Model file for the job. Use its own axes, mm. Coordinates: 2 decimals unless noted, no trailing zeros. Write each loop counter-clockwise with the first axis right and the second up, starting at its lowest first coordinate (ties: lowest second). Pieces come first, ordered by that corner, then holes.
Q1. Band-saw the part on A-A, the plane x = 50. Write the cut outline in (y, z).
Q2. Band-saw the part on B-B, the plane z = 1.75. State how many separate pieces and enclosed holes the cut face has, plus the area to 3 significant figures.
Q3. Drill centre lines: probe 1 along Y at (x, z) = (-70, 2.25); probe 2 along Z at (x, y) = (-20, 6.75); probe 3 along Y at (x, z) = (-70, 6.25). Where is each one in solid material? Low to high.
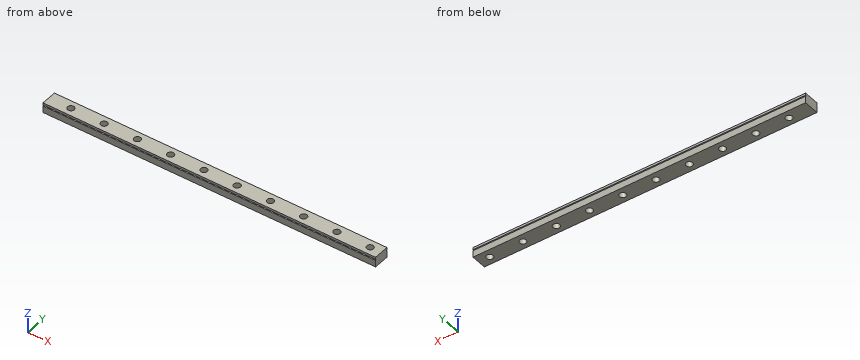
Autodesk Inventor part; units mm, degrees
ref_plane "YZ Plane" through (0, 0, 0) normal (1, 0, 0) x (0, 1, 0)
ref_plane "XZ Plane" through (0, 0, 0) normal (0, 1, 0) x (-1, 0, 0)
ref_plane "XY Plane" through (0, 0, 0) normal (0, 0, 1) x (1, 0, 0)
sketch "Sketch1" plane through (0, 0, 0) normal (0, 0, 1) x (1, 0, 0)
  line L0 (150, -7) -> (-150, -7)
  line L1 (-150, -7) -> (-150, 7)
  line L2 (-150, 7) -> (150, 7)
  line L3 (150, 7) -> (150, -7)
  line L4 (0, 0) -> (0, 3.6651)
  line L5 (0, 0) -> (24.411, 0)
  point P0 (0, 7)
  point P1 (150, 0)
  dimension "d0" = 300
  dimension "d1" = 14
extrude "Extrusion1" add sketch "Sketch1" along normal blind 9
sketch "Sketch2" plane through (-150, -7, 0) normal (-1, 0, 0) x (0, 0, 1)
  line L0 (0, 14) -> (9, 14)
  line L1 (6.5, 13.134) -> (6, 14)
  line L2 (6, 14) -> (7, 14)
  line L3 (7, 14) -> (6.5, 13.134)
  point P0 (0, 7)
  point P1 (6.5, 13.7113)
  dimension "d4" = 1
  dimension "d5" = 2
extrude "Extrusion2" cut sketch "Sketch2" against normal through all
mirror "Mirror1" about plane through (0, 0, 0) normal (0, 1, 0) of "Extrusion2"
sketch "Sketch3" plane through (0, 0, 9) normal (0, 0, 1) x (1, 0, 0)
  line L0 (-150, 7) -> (-150, -7)
  circle A0 centre (-130, 0) radius 3
  point P0 (0, 0)
  dimension "d9" = 6
  dimension "d10" = 20
extrude "Extrusion3" cut sketch "Sketch3" against normal through all
pattern_linear "Rectangular Pattern1" count 10 spacing 30 along (1, 0, 0) of "Extrusion3"
ref_plane "Work Plane1" through (0, 0, 0) normal (0, 1, 0) x (-1, 0, 0)
properties part number "Stand" material "Steel, Wrought"
Answer sheet:
1. outline: (-7, 0) - (-3, 0) - (-3, 9) - (-7, 9) - (-7, 7) - (-6.13, 6.5) - (-7, 6) - close; (3, 0) - (7, 0) - (7, 6) - (6.13, 6.5) - (7, 7) - (7, 9) - (3, 9) - close
2. separate pieces: 1
2. enclosed holes: 10
2. area: 3,920 mm2
3. probe 1: y = -7 to -3, 3 to 7
3. probe 2: z = 0 to 6.14, 6.86 to 9
3. probe 3: y = -6.57 to -3, 3 to 6.57
